Read the model definition and answer for the solid it produces. Units are mm, in the model's axes. Face numbers are marked on the shaded views. A direction names the side the tool comes from. Give positions to 0.01 mm unless a question says otherwise; leave off trailing zeros. Write each loop counter-clockwise with the first axis right and the second up, starting at its lowest first coordinate (ties: lowest second). Pieces come first, ordered by that corner, then holes. Notation, with made-up numbers: (-32, 50) -> (27, 50) arc R23 cw to (27, 88) -> close; hole circle Ø8 at (-8, 56.25). An arc over 180 degrees is marked (long way). Use a Markdown table: item, result.
from build123d import *

# Parameters (mm, degrees)
SKETCH_1_R          = 8
SKETCH_1_R_2        = 5
EXTRUDE_1_DEPTH     = 20
EXTRUDE_2_DEPTH     = 20
SKETCH_3_R          = 1.5
CUT_EXTRUDE_1_DEPTH = 33.496153619
FILLET_1_R          = 2


with BuildPart() as part:
    # 草图1 → 凸台-拉伸1 (new body)
    with BuildSketch(Plane.XY):
        Circle(SKETCH_1_R)
        Circle(SKETCH_1_R_2, mode=Mode.SUBTRACT)
    extrude(amount=EXTRUDE_1_DEPTH)

    # 草图2 → 凸台-拉伸2 (add, through all)
    with BuildSketch(Plane.XY.offset(20)):
        with BuildLine():
            Line((-8, 0), (-8, 20))
            Line((-8, 20), (0, 20))
            Line((0, 20), (0, 8))
            ThreePointArc((0, 8), (-5.656854249, 5.656854249), (-8, 0))
        make_face()
    extrude(amount=-EXTRUDE_2_DEPTH)

    # 草图3 → 切除-拉伸1 (cut, through all)
    with BuildSketch(Plane.ZY.offset(8)):
        with Locations((16, 15)):
            Circle(SKETCH_3_R)
        with BuildLine():
            Line((13.6, 18.2), (0, 8))
            Line((0, 8), (0, 20))
            Line((0, 20), (20, 20))
            Line((20, 20), (20, 15))
            ThreePointArc((20, 15), (17.788854382, 18.577708764), (13.6, 18.2))
        make_face()
    extrude(amount=-CUT_EXTRUDE_1_DEPTH, mode=Mode.SUBTRACT)

    # 圆角1
    # the kernel refuses this fillet: 2 mm, written as the material it adds along each edge
    with BuildSketch(Plane(origin=(0, 8, 20), x_dir=(0.994936153005124, -0.10050896200520786, 0), z_dir=(0, 0, -1))) as fillet_1_piece_1_section:
        with BuildLine():
            CenterArc((1.809161316, -1.989872306), FILLET_1_R, 95.768479516, 78.463040967)
            Line((-0.18071099, -1.788854382), (0, 0))
            ThreePointArc((0, 0), (0.804071696, -0.040510776), (1.608143392, 0))
        make_face()
    fillet_1_piece_1 = extrude(amount=20, mode=Mode.PRIVATE)
    fillet_1_piece_1 = split(fillet_1_piece_1, bisect_by=Plane(origin=(0.363016692, 13.065708847, 6.754278462), z_dir=(0, -0.8000000000000002, 0.5999999999999999)), keep=Keep.TOP, mode=Mode.PRIVATE)
    add(fillet_1_piece_1)


solid = part.part
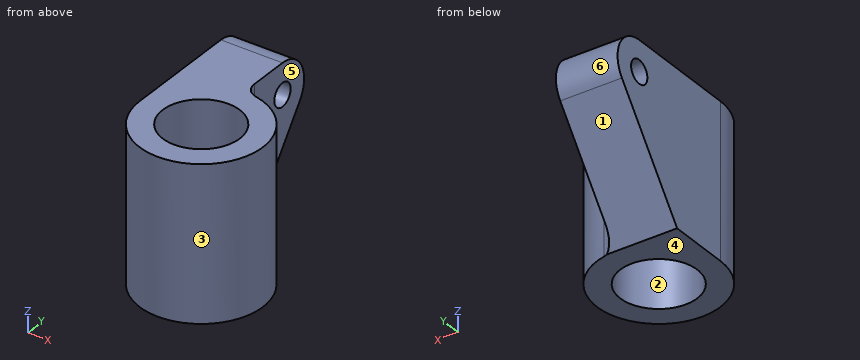
Item 1: This flat-tipped pin is pushed along its axis until it touches: P1, Ø3, axis at y = 15.5, z = 10, coming from the +X side. Where does it stop, or does it pass through?
Return value:
| item | result |
|---|---|
| P1 | x = 0 |
Item 2: A tool of negligible diameter and unlimited length cuts with its end or side. For the marked faces 5 and 6, from which of +Z, -Z, +X, -X, +Y, -Y can it reach the whole face along a straight path? Write none if from no direction.
Return value:
| item | result |
|---|---|
| face 5 | +Z, -Z, +X, +Y |
| face 6 | +X, -X, +Y |
Item 3: A cutting plane is placed at A-A (z = 16). Give the vertices of the cut face in (x, y).
Return value:
| item | result |
|---|---|
| outline | (-8, 0) arc R8 ccw (long way) to (1.6, 7.84) arc R2 cw to (0, 9.8) -> (0, 13.5) -> (-8, 13.5) -> close; (-8, 16.5) -> (0, 16.5) -> (0, 19) -> (-8, 19) -> close; hole circle Ø10 at (0, 0) |
Item 4: Straight lines are drawn through the part: line 1 along X through (y, z) = (-0.25, 5.75); line 2 along X through (y, z) = (16.25, 12); line 3 along Y through (x, z) = (-3.5, 15). For each, find the intervals that lie inside material, in ascending order. Write a range as [from, to].
Return value:
| item | result |
|---|---|
| line 1 | [-8, -4.99], [4.99, 8] |
| line 2 | [-8, 0] |
| line 3 | [-7.19, -3.57], [3.57, 13.88], [16.12, 18.87] |
Item 5: A cutting plane is placed at B-B (z = 6). Give the vertices of the cut face in (x, y), then the cut area to 3 significant figures.
Return value:
| item | result |
|---|---|
| outline | (-8, 0) arc R8 ccw (long way) to (1.6, 7.84) arc R2 cw to (0, 9.8) -> (0, 12.5) -> (-8, 12.5) -> close; hole circle Ø10 at (0, 0) |
| area | 173 mm^2 |
Item 6: A cutting plane is placed at D-D (y = 10.25). Give the vertices of the cut face in (x, z).
Return value:
| item | result |
|---|---|
| outline | (-8, 3) -> (0, 3) -> (0, 20) -> (-8, 20) -> close |
Item 7: For a pull along Y with two mould halves and no side action, classify the marked faces 1, 2, 3 and 4 as +Y half, -Y half, draft (parallel to the pull), parting line (faces both ways), or undercut.
Return value:
| item | result |
|---|---|
| face 1 | +Y half |
| face 2 | undercut |
| face 3 | parting line |
| face 4 | draft |
Item 8: A cutting plane is placed at C-C (y = -1.75). Give the vertices of the cut face in (x, z), then the cut area to 3 significant figures.
Return value:
| item | result |
|---|---|
| outline | (-7.81, 0) -> (-4.68, 0) -> (-4.68, 20) -> (-7.81, 20) -> close; (4.68, 0) -> (7.81, 0) -> (7.81, 20) -> (4.68, 20) -> close |
| area | 125 mm^2 |
